The listing builds one solid part. Answer for the finished solid, in the listing's coordinates (mm). Face numbers are marked on the shaded views. A direction names the side the tool comes from. Round coordinates to 2 decimals unless told otherwise and drop trailing zeros. Write each loop counter-clockwise with the first axis right and the second up, starting at its lowest first coordinate (ties: lowest second). Pieces come first, ordered by that corner, then holes. Notation, with made-up numbers: (-33.5, 52) - (-18.5, 52) arc R19 ccw to (-18.5, 88) - close; hole circle Ø8 at (74.5, 20). An arc over 180 degrees is marked (long way). Answer as CSV lines item,"result". Start each with the question number.
Item 1: Straight lines are drawn through the part: line 1 along Y through (x, z) = (0, 35.5); line 2 along X through (y, z) = (-25, 21) (3 decimals); line 3 along Y through (x, z) = (2, 11.5). For each, find the intervals that lie inside material, in ascending order. Write a range as [from, to].
Item 2: For a pull along X with two mould halves and no side action, classify the marked faces 3, 4 and 5 as pulls with the +X half, pulls with the -X half, needs draft (parallel to the pull), parting line crosses it, or undercut.
Item 3: A cutting plane is placed at D-D on x = -12. Determine the outline of the cut face in (y, z).
Item 4: A cutting plane is placed at A-A on x = 0. Determine the outline of the cut face in (y, z), and give its area (3 significant figures).
Item 5: A cutting plane is placed at C-C on z = 47.5. Determine the outline of the cut face in (x, y) (3 decimals).
Item 6: Which of the six approach directions +Z, -Z, +X, -X, +Y, -Y give full straight-line access (tool end or side, diameter ignored) to the marked faces 1 and 2?
Item 7: Flat-ended cylindrical pins translate along their axes: pin 1 (8.5 mm diameter, centred on x = 0, y = -25.4, fed in from +Z); pin 2 (6.5 mm diameter, centred on x = 1.5, y = -22.5, fed in from -Z). Find the tip coordinate at first contact, or state that the pin passes through.
```python
from build123d import *

# Parameters (mm, degrees)
BASE_EXTRUDE_DEPTH               = 15.875
F_1_2_13_TAPPED_HOLE2_AT_2_COUNT = 2
F_1_2_13_TAPPED_HOLE2_AT_2_PITCH = 50.8


with BuildPart() as part:
    # Sketch1 → Base-Extrude (new, symmetric)
    with BuildSketch(Plane(origin=(0, 0, 0), x_dir=(0, 0, -1), z_dir=(1, 0, 0))):
        with BuildLine():
            Line((-50.8, 44.45), (-50.8, -44.45))
            Line((-50.8, -44.45), (-1.5875, -44.45))
            Line((-1.5875, -44.45), (-1.5875, -16.050684869))
            ThreePointArc((-1.5875, -16.050684869), (-16.129, 0), (-1.5875, 16.050684869))
            Line((-1.5875, 16.050684869), (-1.5875, 44.45))
            Line((-1.5875, 44.45), (-50.8, 44.45))
        make_face()
    extrude(amount=BASE_EXTRUDE_DEPTH, both=True)

    # Sketch6 → 1/2-13 Tapped Hole2 (revolve, cut)
    with BuildSketch(Plane(origin=(0, 25.4, 1.5875), x_dir=(0, 1, 0), z_dir=(1, 0, 0))):
        Polygon((0, 0), (0, 49.2125), (5.35813, 49.2125), (5.35813, 25.4), (6.35, 25.4), (6.35, 0.79375), (7.14375, 0), align=None)
    f_1_2_13_tapped_hole2 = revolve(axis=Axis((0, 25.4, -4.7625), (0, 0, 1)), mode=Mode.SUBTRACT)

    # 1/2-13 Tapped Hole2 at 2: 1/2-13 Tapped Hole2 ×2
    with Locations(*[(0, -i * F_1_2_13_TAPPED_HOLE2_AT_2_PITCH, 0) for i in range(1, F_1_2_13_TAPPED_HOLE2_AT_2_COUNT)]):
        add(f_1_2_13_tapped_hole2, mode=Mode.SUBTRACT)


solid = part.part
```
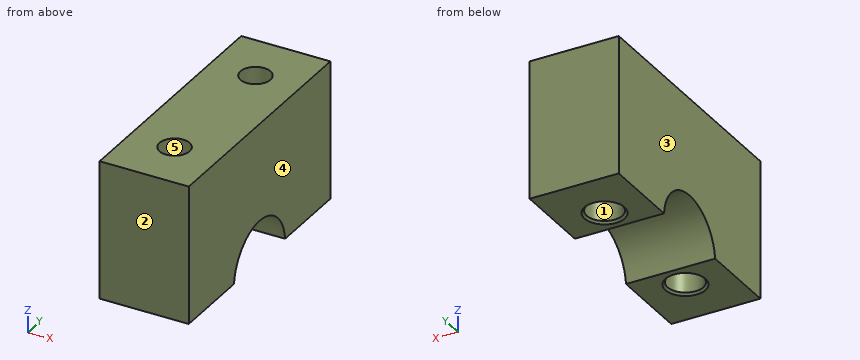
Geometry says:
1,line 1,"y = [-44.45, -30.76], [-20.04, 20.04], [30.76, 44.45]"
1,line 2,"x = [-15.875, -6.337], [6.337, 15.875]"
1,line 3,"y = [-44.45, -31.43], [-19.37, -11.31], [11.31, 19.37], [31.43, 44.45]"
2,face 3,"pulls with the -X half"
2,face 4,"pulls with the +X half"
2,face 5,"undercut"
3,outline,"(-44.45, 1.59) - (-16.05, 1.59) arc R16.13 cw to (16.05, 1.59) - (44.45, 1.59) - (44.45, 50.8) - (-44.45, 50.8) - close"
4,outline,"(-44.45, 1.59) - (-32.54, 1.59) - (-31.75, 2.38) - (-31.75, 26.99) - (-30.76, 26.99) - (-30.76, 50.8) - (-44.45, 50.8) - close; (-20.04, 26.99) - (-19.05, 26.99) - (-19.05, 2.38) - (-18.26, 1.59) - (-16.05, 1.59) arc R16.13 cw to (16.05, 1.59) - (18.26, 1.59) - (19.05, 2.38) - (19.05, 26.99) - (20.04, 26.99) - (20.04, 50.8) - (-20.04, 50.8) - close; (30.76, 26.99) - (31.75, 26.99) - (31.75, 2.38) - (32.54, 1.59) - (44.45, 1.59) - (44.45, 50.8) - (30.76, 50.8) - close"
4,area,"2,860 mm^2"
5,outline,"(-15.875, -44.45) - (15.875, -44.45) - (15.875, 44.45) - (-15.875, 44.45) - close; hole circle Ø10.716 at (0, -25.4); hole circle Ø10.716 at (0, 25.4)"
6,face 1,"-Z"
6,face 2,"+Z, -Z, +X, -X, -Y"
7,pin 1,"passes through"
7,pin 2,"stops at z = 2.22"
